Here's how the part is built. I have some questions about the finished solid (model axes, mm). Give positions to 0.01 mm unless a question says otherwise; leave off trailing zeros. Order: outer loops, then holes, each group sorted by start corner. A loop starts at its lowest first (then second) coordinate and runs counter-clockwise, first axis right, second up. Notation, with made-up numbers: M 26.25,21 L 57.25,21 A8 cw 57.25,33 Z; hole C 82,-21.75 d7. An arc over 180 degrees is marked long. Use one line per item in the form item = value.
from build123d import *

# Parameters (mm, degrees)
ESQUISSE1_R             = 14.5
BOSS_EXTRU_1_DEPTH      = 41
ESQUISSE2_R             = 12.95
BOSS_EXTRU_2_DEPTH      = 3.4
BOSS_EXTRU_3_DEPTH      = 6
BOSS_EXTRU_3_DEPTH_BACK = 1
ESQUISSE3_W             = 0.8
ESQUISSE3_H             = 2.4
BOSS_EXTRU_4_DEPTH      = 6
BOSS_EXTRU_4_DEPTH_BACK = 1
ESQUISSE4_W             = 0.8
ESQUISSE4_H             = 2.4
CONG_1_R                = 1.2


with BuildPart() as part:
    # Esquisse1 → Boss.-Extru.1 (new body)
    with BuildSketch(Plane.XY):
        Circle(ESQUISSE1_R)
    extrude(amount=BOSS_EXTRU_1_DEPTH)

    # Esquisse2 → Boss.-Extru.2 (add)
    with BuildSketch(Plane(origin=(0, 0, 0), x_dir=(-1, 0, 0), z_dir=(0, 0, -1))):
        with Locations(Location((0, 0, 0), (0, 0, 180))):
            Circle(ESQUISSE2_R)
    extrude(amount=BOSS_EXTRU_2_DEPTH)

    # Esquisse3 → Boss.-Extru.3 (add, two sides: drawn at the far end of the back side and taken through both)
    with BuildSketch(Plane(origin=(12.95, 0, 0), x_dir=(0, 0, -1), z_dir=(1, 0, 0)).offset(-BOSS_EXTRU_3_DEPTH_BACK)):
        with Locations((2.4, 0)):
            Rectangle(ESQUISSE3_W, ESQUISSE3_H)
    extrude(amount=BOSS_EXTRU_3_DEPTH + BOSS_EXTRU_3_DEPTH_BACK)

    # Esquisse4 → Boss.-Extru.4 (add, two sides: drawn at the far end of the back side and taken through both)
    with BuildSketch(Plane.ZY.offset(12.95).offset(-BOSS_EXTRU_4_DEPTH_BACK)):
        with Locations((-2.4, 0)):
            Rectangle(ESQUISSE4_W, ESQUISSE4_H)
    extrude(amount=BOSS_EXTRU_4_DEPTH + BOSS_EXTRU_4_DEPTH_BACK)

    # Congé1
    cong_1_edges = [part.edges().sort_by_distance(p)[0] for p in [
        (18.95, -1.2, -2.4),
        (18.95, 1.2, -2.4),
        (-18.95, -1.2, -2.4),
        (-18.95, 1.2, -2.4),
    ]]
    fillet(cong_1_edges, radius=CONG_1_R - 0.0001)  # a hair under: the kernel refuses the full size


solid = part.part
Q1. I'm going to push flat-ended pins straight in: pin 1 Ø0.6 at (x, z) = (-14.5, -2.5) entering from +Y; pin 2 Ø3 at (y, z) = (-1, 4) entering from +X; pin 3 Ø1.2 at (x, y) = (-15.5, -0.5) entering from -Z; pin 4 Ø6 at (x, z) = (-0.5, 1.5) entering from -Y. Where does each tip first touch, or does it pass through?
Found:
pin_1 = 1.2
pin_2 = 14.5
pin_3 = -2.8
pin_4 = -14.5
Q2. I want a section at B-B on y = 5.5. Write out the boundary of the cut face in (x, z), then the cut area to 3 significant figures.
Found:
outline = M -13.42,0 L -11.72,0 L -11.72,-3.4 L 11.72,-3.4 L 11.72,0 L 13.42,0 L 13.42,41 L -13.42,41 Z
area = 1,180 mm²
Q3. I want a section at A-A on x = 5. Write out the boundary of the cut face in (y, z).
Found:
outline = M -13.61,0 L -11.95,0 L -11.95,-3.4 L 11.95,-3.4 L 11.95,0 L 13.61,0 L 13.61,41 L -13.61,41 Z
Q4. Thinking about a two-plate mould opening in Z: for faces 1 (the face through (-18.608, -0.839, -2.394)), 2 (the face through (16, 0, -2.8)), 3 (the face through (16, 0, -2)), which applies, +Z half, -Z half, draft (parallel to the pull), parting line (faces both ways), or undercut?
Found:
face_1 = draft
face_2 = -Z half
face_3 = undercut
Q5. I need wall thicknesses on L1, parallel to Z at x = -16.5, y = -0.5; L2, parallel to Z at x = 13, y = -4; L3, parallel to Y at x = 4, z = 33. Which ranges of each line are inside material? Lowest first, please.
Found:
L1 = -2.8 to -2
L2 = 0 to 41
L3 = -13.94 to 13.94
Q6. I want a section at C-C on z = 36. Write out the boundary of the cut face in (x, y), then the cut area to 3 significant figures.
Found:
outline = C 0,0 d29
area = 661 mm²
Q7. I want a section at D-D on x = -15.5. Write out the boundary of the cut face in (y, z), then the cut area to 3 significant figures.
Found:
outline = M -1.2,-2.8 L 1.2,-2.8 L 1.2,-2 L -1.2,-2 Z
area = 1.92 mm²
